CAD build for the part. Positions are in the model's coordinates, mm. Face numbers are marked on the shaded views. A direction names the side the tool comes from. Give positions to 0.01 mm unless a question says otherwise; leave off trailing zeros. Loops run counter-clockwise (first coordinate to the right, second up) from the corner with the lowest first, then second, coordinate; pieces in that order, holes last. Notation, with made-up numbers: (-27, 38.5) - (-20, 38.5) arc R22 cw to (-20, 51.5) - close; hole circle Ø5 at (40.25, 55.5). An arc over 180 degrees is marked (long way). Return JSON: item names as keys, results as strings.
from build123d import *

# Parameters (mm, degrees)
SKETCH1_W                          = 50
SKETCH1_H                          = 40
BOSS_EXTRUDE1_DEPTH                = 4
SKETCH2_W                          = 7.705962758
SKETCH2_H                          = 14.539090136
CUT_EXTRUDE1_DEPTH                 = 122.811546491
SKETCH3_W                          = 10.372123492
SKETCH3_H                          = 14.267331442
CUT_EXTRUDE2_DEPTH                 = 122.811546491
F_2_0_2_DIAMETER_HOLE1_D           = 2
F_2_0_2_DIAMETER_HOLE1_CSINK_D     = 8
F_2_0_2_DIAMETER_HOLE1_CSINK_ANGLE = 90


with BuildPart() as part:
    # Sketch1 → Boss-Extrude1 (new body)
    with BuildSketch(Plane(origin=(0, 0, 34.811611197), x_dir=(-1, 0, 0), z_dir=(0, 0, -1))):
        with Locations((1.46446617, 98.834695645)):
            Rectangle(SKETCH1_W, SKETCH1_H)
    extrude(amount=-BOSS_EXTRUDE1_DEPTH)

    # Sketch2 → Cut-Extrude1 (cut, through all)
    with BuildSketch(Plane.XY.offset(38.811611197)):
        with Locations((19.682552451, 98.267628733)):
            Rectangle(SKETCH2_W, SKETCH2_H)
    extrude(amount=-CUT_EXTRUDE1_DEPTH, mode=Mode.SUBTRACT)

    # Sketch3 → Cut-Extrude2 (cut, through all)
    with BuildSketch(Plane.XY.offset(38.811611197)):
        with Locations((1.539593072, 98.131749386)):
            Rectangle(SKETCH3_W, SKETCH3_H)
    extrude(amount=-CUT_EXTRUDE2_DEPTH, mode=Mode.SUBTRACT)

    # Ø2.0 (2) Diameter Hole1 (through all)
    with Locations(Plane(origin=(0, 0, 34.811611197), x_dir=(-1, 0, 0), z_dir=(0, 0, -1))):
        with Locations((-3.156646479, 84.016340669), (-19.156646479, 84.016340669), (-19.156646479, 114.016340669), (-3.156646479, 114.016340669)):
            CounterSinkHole(F_2_0_2_DIAMETER_HOLE1_D / 2, F_2_0_2_DIAMETER_HOLE1_CSINK_D / 2, counter_sink_angle=F_2_0_2_DIAMETER_HOLE1_CSINK_ANGLE)


solid = part.part
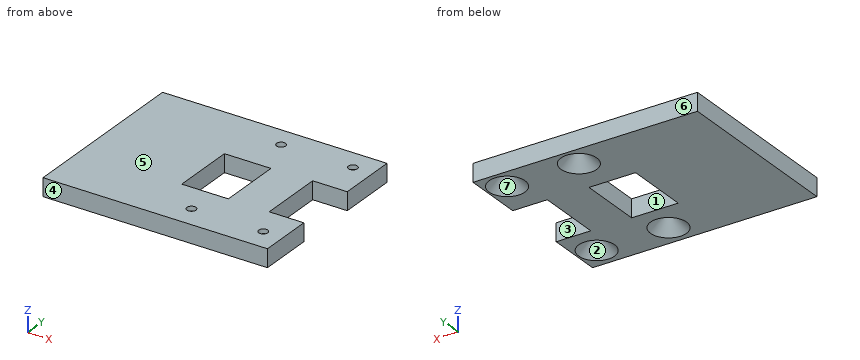
1. Cut at B-B, the plane z = 35.75. Write the cut outline in (x, y).
Values follow:
{"outline": "(-26.46, 78.83) - (23.54, 78.83) - (23.54, 91) - (15.83, 91) - (15.83, 105.54) - (23.54, 105.54) - (23.54, 118.83) - (-26.46, 118.83) - close; hole (-3.65, 91) - (6.73, 91) - (6.73, 105.27) - (-3.65, 105.27) - close; hole circle Ø6.12 at (3.16, 84.02); hole circle Ø6.12 at (3.16, 114.02); hole circle Ø6.12 at (19.16, 84.02); hole circle Ø6.12 at (19.16, 114.02)"}
2. Drill centre lines: probe 1 along X at (y, z) = (96, 35.1); probe 2 along Y at (x, z) = (16.5, 37.4); probe 3 along X at (y, z) = (116, 35.1). Where is each one in solid material? Low to high.
Values follow:
{"probe 1": "x = -26.46 to -3.65, 6.73 to 15.83", "probe 2": "y = 78.83 to 91, 105.54 to 118.83", "probe 3": "x = -26.46 to 0.02, 6.29 to 16.02, 22.29 to 23.54"}
3. Which spindle directions (+Z, -Z, +X, -X, +Y, -Y) get a long thin tool onto all of the face, cutting with end or side? Do the marked faces 1, 2 and 3. Say none if no direction does.
Values follow:
{"face 1": "+Z, -Z", "face 2": "-Z", "face 3": "+Z, -Z, +X"}
4. Pull direction Y, two halves, no side cores. Call the marked faces 4, 5, 6 and 7: +Y half, -Y half, draft (parallel to the pull), parting line (faces both ways), or undercut.
Values follow:
{"face 4": "-Y half", "face 5": "draft", "face 6": "+Y half", "face 7": "undercut"}
5. Cut at A-A, the plane y = 95. Write the cut outline in (x, z), plus the area to 3 significant figures.
Values follow:
{"outline": "(-26.46, 34.81) - (-3.65, 34.81) - (-3.65, 38.81) - (-26.46, 38.81) - close; (6.73, 34.81) - (15.83, 34.81) - (15.83, 38.81) - (6.73, 38.81) - close", "area": "128 mm²"}
6. Drop flat-ended pins along their axis: P1, Ø3, axis at x = 19.16, y = 114.02, coming from the +Z side; P2, Ø1.2, axis at y = 98, z = 37.5, coming from the +X side; P3, Ø2.5, axis at x = 3.16, y = 84.02, coming from the -Z side. Give the stop position or say it passes through.
Values follow:
{"P1": "stops at z = 38.81", "P2": "stops at x = 15.83", "P3": "stops at z = 37.56"}
